Input: part model. Units: mm. Frame: model coordinates. Face numbers are marked on the shaded views. A direction names the side the tool comes from. Round coordinates to 2 decimals unless told otherwise and drop trailing zeros. Loops run counter-clockwise (first coordinate to the right, second up) from the corner with the lowest first, then second, coordinate; pieces in that order, holes last. Notation, with made-up numbers: (30, -7) -> (38, -7) arc R15 ccw to (38, 20) -> close; hole circle Ø2 at (1.5, -18). An arc over 180 degrees is marked (long way). Answer as a JSON object with one key per item and string values. Group by question number.
Item 1: Section query C-C on z = 4.75. Return loops of the section in (x, y).
Item 2: Section query B-B on x = 40.5. Return loops of the section in (y, z).
Item 3: Section query A-A on y = -55.5. Return loops of the section in (x, z).
Item 4: Material intervals for line 1 (X direction, y = -34, z = 13.5); line 2 (X direction, y = -31.1, z = 12.5); line 3 (X direction, y = -50, z = 13.25), sorted ascending. Write a range as [from, to].
Item 5: Section query D-D on z = 20.95. Count the separate pieces of the cut face and the enclosed holes in it, and give its area (3 significant figures).
Item 6: Pin query (flat end, axial travel): pin 1 (4 mm diameter, centred on x = 10.5, z = 12.5, fed in from +Y); pin 2 (5 mm diameter, centred on x = 50.5, y = -53, fed in from -Z); pin 3 (8 mm diameter, centred on y = -49.5, z = 21, fed in from +X); pin 4 (5 mm diameter, centred on x = 70.5, y = -36, fed in from +Z). Return the tip coordinate at first contact, or that it passes through.
Item 7: Set-up query: the marked faces 1, 2 and 3. Return all of +Z, -Z, +X, -X, +Y, -Y with unobstructed straight access to the full face (end or side cutting, diameter ignored); none if empty.
Item 8: Draft query along X for the marked faces 4, 5, 6 and 7. Return one class per face: released by +X, released by -X, zero draft, split by the parting line, or undercut.
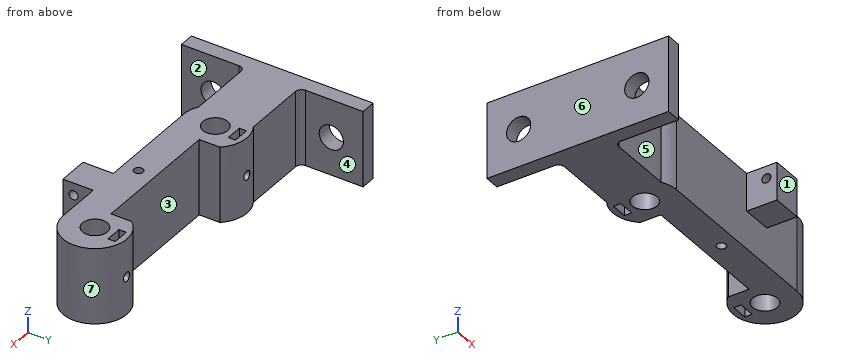
from build123d import *

# Parameters (mm, degrees)
SKETCH005_R          = 4.1
PAD004_DEPTH         = 25
SKETCH010_W          = 44
SKETCH010_H          = 50
POCKET003_DEPTH      = 25
PAD008_DEPTH         = 25
SKETCH018_W          = 10
SKETCH018_H          = 12.5
SKETCH018_R          = 1.5
PAD009_DEPTH         = 10
SKETCH019_R          = 1.5
POCKET009_DEPTH      = 0.001
POCKET009_DEPTH_BACK = 25.001
SKETCH020_W          = 5.5
SKETCH020_H          = 2.4
POCKET010_DEPTH      = 0.001
POCKET010_DEPTH_BACK = 25.001
SKETCH021_R          = 1.5
POCKET011_DEPTH      = 30.001
SKETCH043_R          = 4
POCKET027_DEPTH      = 22.9093269132
FILLET_R             = 2


with BuildPart() as part:
    # Sketch005 → Pad004 (new body)
    with BuildSketch(Plane.XY):
        with BuildLine():
            ThreePointArc((21, 0), (3.0753787975, 7.4246212025), (10.5, -10.5))
            Line((10.5, -10.5), (70.5, -10.5))
            ThreePointArc((70.5, -10.5), (77.9246212025, 7.4246212025), (60, 0))
            Line((21, 0), (60, 0))
        make_face()
        with Locations((10.5, 0)):
            Circle(SKETCH005_R, mode=Mode.SUBTRACT)
        with Locations((70.5, 0)):
            Circle(SKETCH005_R, mode=Mode.SUBTRACT)
    extrude(amount=PAD004_DEPTH)

    # Sketch010 → Pocket003 (cut)
    with BuildSketch(Plane.XY):
        with Locations((40.5, 25)):
            Rectangle(SKETCH010_W, SKETCH010_H)
    extrude(amount=POCKET003_DEPTH, mode=Mode.SUBTRACT)

    # Sketch017 → Pad008 (join)
    with BuildSketch(Plane.XY):
        with BuildLine():
            Line((5.0916730868, 9), (-17.9083269132, 9))
            Line((-17.9083269132, 30), (-17.9083269132, 9))
            Line((-22.9083269132, 30), (-17.9083269132, 30))
            Line((-22.9083269132, -30), (-22.9083269132, 30))
            Line((-17.9083269132, -30), (-22.9083269132, -30))
            Line((-17.9083269132, -9), (-17.9083269132, -30))
            Line((-17.9083269132, -9), (5.0916730868, -9))
            ThreePointArc((5.0916730868, 9), (0, 0), (5.0916730868, -9))
        make_face()
    extrude(amount=PAD008_DEPTH)

    # Sketch018 → Pad009 (join)
    with BuildSketch(Plane.YZ.offset(45.51)):
        with Locations((-15.5, 18.75)):
            Rectangle(SKETCH018_W, SKETCH018_H)
        with Locations((-17, 20.95)):
            Circle(SKETCH018_R, mode=Mode.SUBTRACT)
    extrude(amount=PAD009_DEPTH)

    # Sketch019 → Pocket009 (cut, two sides)
    with BuildSketch(Plane.XY) as pocket009_sk:
        with Locations((40.5, -5.45)):
            Circle(SKETCH019_R)
    extrude(amount=-POCKET009_DEPTH, mode=Mode.SUBTRACT)
    extrude(pocket009_sk.sketch, amount=POCKET009_DEPTH_BACK, mode=Mode.SUBTRACT)

    # Sketch020 → Pocket010 (cut, two sides)
    with BuildSketch(Plane.XY) as pocket010_sk:
        with Locations((10.5, 7.3)):
            Rectangle(SKETCH020_W, SKETCH020_H)
        with Locations((70.5, 7.3)):
            Rectangle(SKETCH020_W, SKETCH020_H)
    extrude(amount=-POCKET010_DEPTH, mode=Mode.SUBTRACT)
    extrude(pocket010_sk.sketch, amount=POCKET010_DEPTH_BACK, mode=Mode.SUBTRACT)

    # Sketch021 → Pocket011 (cut, through all)
    with BuildSketch(Plane.XZ):
        with Locations((10.5, 12.5)):
            Circle(SKETCH021_R)
        with Locations((70.5, 12.5)):
            Circle(SKETCH021_R)
    extrude(amount=-POCKET011_DEPTH, mode=Mode.SUBTRACT)

    # Sketch043 → Pocket027 (cut, through all)
    with BuildSketch(Plane.YZ):
        with Locations((-19.5, 12.5)):
            Circle(SKETCH043_R)
        with Locations((19.5, 12.5)):
            Circle(SKETCH043_R)
    extrude(amount=-POCKET027_DEPTH, mode=Mode.SUBTRACT)

    # Fillet
    fillet_edges = [part.edges().sort_by_distance(p)[0] for p in [
        (-17.908327, 9, 12.5),
        (-17.908327, -9, 12.5),
    ]]
    fillet(fillet_edges, radius=FILLET_R)


with BuildPart() as part_1:
    # Body004 placement: moved
    add(part.part.moved(Location((0, -36, 0))))


solid = part_1.part
Solved:
{
 "1": {"outline": "(-22.91, -66) -> (-17.91, -66) -> (-17.91, -47) arc R2 cw to (-15.91, -45) -> (5.09, -45) arc R10.5 ccw to (10.5, -46.5) -> (70.5, -46.5) arc R10.5 ccw (long way) to (62.5, -29.2) -> (62.5, -36) -> (18.5, -36) -> (18.5, -29.2) arc R10.5 ccw to (5.09, -27) -> (-15.91, -27) arc R2 cw to (-17.91, -25) -> (-17.91, -6) -> (-22.91, -6) -> close; hole circle Ø8.2 at (10.5, -36); hole (7.75, -29.9) -> (13.25, -29.9) -> (13.25, -27.5) -> (7.75, -27.5) -> close; hole circle Ø3 at (40.5, -41.45); hole circle Ø8.2 at (70.5, -36); hole (67.75, -29.9) -> (73.25, -29.9) -> (73.25, -27.5) -> (67.75, -27.5) -> close"},
 "2": {"outline": "(-46.5, 0) -> (-42.95, 0) -> (-42.95, 25) -> (-46.5, 25) -> close; (-39.95, 0) -> (-36, 0) -> (-36, 25) -> (-39.95, 25) -> close"},
 "3": {"outline": "(-22.91, 0) -> (-17.91, 0) -> (-17.91, 8.5) -> (-22.91, 8.5) -> close; (-22.91, 16.5) -> (-17.91, 16.5) -> (-17.91, 25) -> (-22.91, 25) -> close; (45.51, 12.5) -> (55.51, 12.5) -> (55.51, 25) -> (45.51, 25) -> close"},
 "4": {"line 1": "[-22.91, 6.92], [14.08, 18.5], [62.5, 66.92], [74.08, 80.81]", "line 2": "[-22.91, 9], [12, 18.5], [62.5, 69], [72, 79.79]", "line 3": "[-22.91, -17.91], [45.51, 55.51]"},
 "5": {"separate pieces": "2", "enclosed holes": "5", "area": "1,710 mm²"},
 "6": {"pin 1": "y = -25.5", "pin 2": "z = 12.5", "pin 3": "x = 74.97", "pin 4": "through"},
 "7": {"face 1": "+Z, -Z, +X, -Y", "face 2": "+Z, -Z, -Y", "face 3": "+Z, -Z, +Y"},
 "8": {"face 4": "released by +X", "face 5": "undercut", "face 6": "released by -X", "face 7": "undercut"}
}
